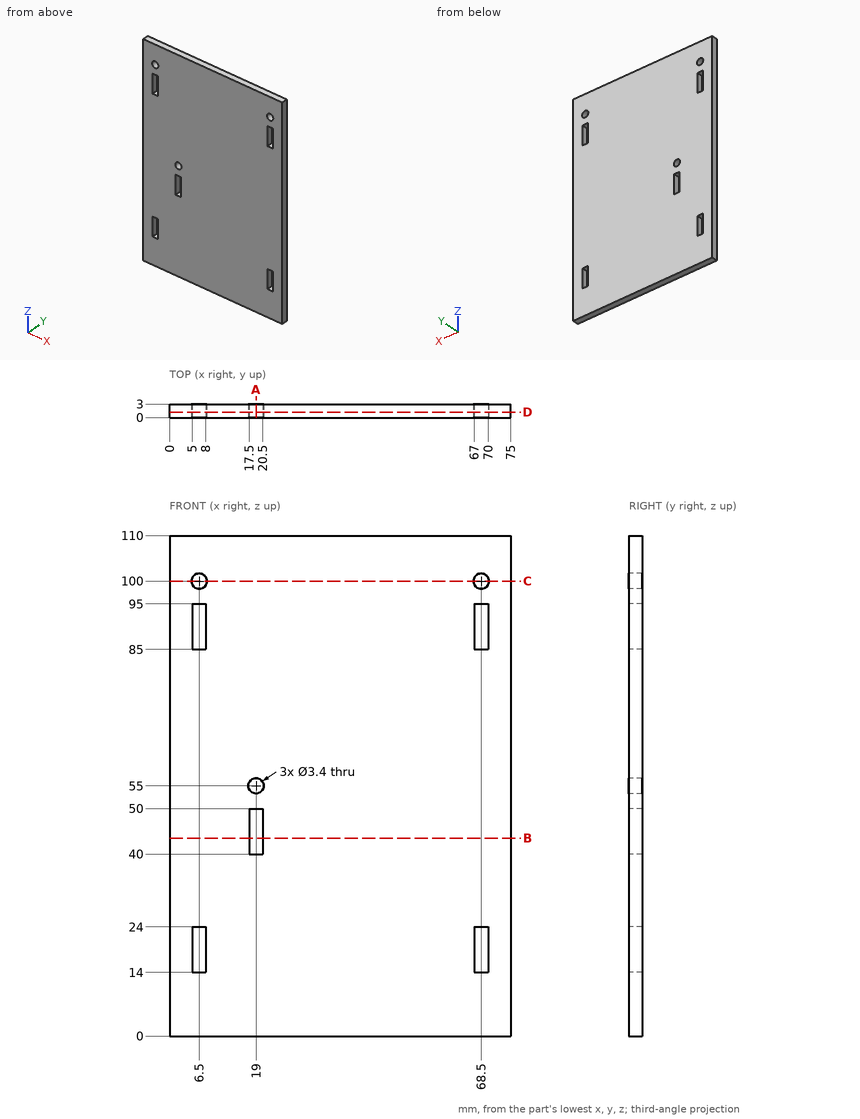
The figure shows three views and two pictorial views of one solid part (mm, origin at its lowest corner). Answer the questions. Round coordinates to 2 decimals unless told otherwise and drop trailing zeros. Write each loop counter-clockwise with the first axis right and the second up, starting at its lowest first coordinate (ties: lowest second). Pieces come first, ordered by that corner, then holes. Notation, with made-up numbers: M 84,-29 L 126,-29 A17 ccw 126,-18 Z; hole C -7.5,51.5 d9. An arc over 180 degrees is marked long. Use a Markdown table: item, result.
1) The part is cut by section C-C on z = 100. Give the vertices of the cut face in (x, y).
Taken from the geometry:
| item | result |
|---|---|
| outline | M 0,0 L 4.8,0 L 4.8,3 L 0,3 Z; M 8.2,0 L 66.8,0 L 66.8,3 L 8.2,3 Z; M 70.2,0 L 75,0 L 75,3 L 70.2,3 Z |
2) Consider line 1 (Z direction, x = 68.5, y = 2.1); line 2 (X direction, y = 1.5, z = 100); line 3 (X direction, y = 1.6, z = 55). Determine where each line is inside the solid, lowest interval first. Write a range as [from, to].
Taken from the geometry:
| item | result |
|---|---|
| line 1 | z = [0, 14], [24, 85], [95, 98.3], [101.7, 110] |
| line 2 | x = [0, 4.8], [8.2, 66.8], [70.2, 75] |
| line 3 | x = [0, 17.3], [20.7, 75] |
3) The part is cut by section D-D on y = 1.2. State how many separate pieces and enclosed holes the cut face has, plus the area to 3 significant figures.
Taken from the geometry:
| item | result |
|---|---|
| separate pieces | 1 |
| enclosed holes | 8 |
| area | 8,070 mm2 |
4) The part is cut by section B-B on z = 43.5. Give the vertices of the cut face in (x, y).
Taken from the geometry:
| item | result |
|---|---|
| outline | M 0,0 L 17.5,0 L 17.5,3 L 0,3 Z; M 20.5,0 L 75,0 L 75,3 L 20.5,3 Z |
5) The part is cut by section A-A on x = 19. Give the vertices of the cut face in (y, z).
Taken from the geometry:
| item | result |
|---|---|
| outline | M 0,0 L 3,0 L 3,40 L 0,40 Z; M 0,50 L 3,50 L 3,53.3 L 0,53.3 Z; M 0,56.7 L 3,56.7 L 3,110 L 0,110 Z |
6) A flat-ended cylindrical pin translates along its axis: pin 1 (2 mm diameter, centred on x = 68.5, z = 100, fed in from +Y). Find the tip coordinate at first contact, or state that the pin passes through.
Taken from the geometry:
| item | result |
|---|---|
| pin 1 | passes through |
